The model under review builds one solid part; all positions refer to its coordinate system, in mm. A direction names the side the tool comes from. Round coordinates to 2 decimals unless told otherwise and drop trailing zeros. Write each loop counter-clockwise with the first axis right and the second up, starting at its lowest first coordinate (ties: lowest second). Pieces come first, ordered by that corner, then holes. Notation, with made-up numbers: (38, 45.25) -> (75, 45.25) arc R8 ccw to (75, 52.25) -> close; hole circle Ø7 at (25.25, 28.25). An arc over 180 degrees is marked (long way). Answer in a Markdown table with one row per item. Add a question column.
```python
from build123d import *

# Parameters (mm, degrees)
F0_W      = 77
F0_H      = 91
F0_W_2    = 50
F0_H_2    = 85
F1_DEPTH  = 3.1
F2_W      = 77
F2_H      = 91
F2_W_2    = 71
F2_H_2    = 85
F3_DEPTH  = 5
F4_W      = 3
F4_H      = 91
F5_DEPTH  = 25
F6_W      = 77
F6_H      = 91
F6_W_2    = 71
F6_H_2    = 85
F7_DEPTH  = 70
F9_DEPTH  = 91
F11_DEPTH = 77
F12_W     = 6
F12_H     = 8.1
F13_DEPTH = 4
F15_DEPTH = 91
F16_W     = 3
F16_H     = 91
F17_DEPTH = 25
F18_R     = 3


with BuildPart() as f1:
    # F0 (on Top) → F1 (new body)
    with BuildSketch(Plane.XY):
        Rectangle(F0_W, F0_H)
        Rectangle(F0_W_2, F0_H_2, mode=Mode.SUBTRACT)
    extrude(amount=F1_DEPTH)

    # F2 (on face) → F3 (join)
    with BuildSketch(Plane.XY.offset(3.1)):
        Rectangle(F2_W, F2_H)
        Rectangle(F2_W_2, F2_H_2, mode=Mode.SUBTRACT)
    extrude(amount=F3_DEPTH)

    # F4 (on face) → F5 (join)
    with BuildSketch(Plane.XY.offset(8.1)):
        with Locations((-37, 0)):
            Rectangle(F4_W, F4_H)
        with Locations((37, 0)):
            Rectangle(F4_W, F4_H)
    extrude(amount=F5_DEPTH)

    # F6 (on face) → F7 (join)
    with BuildSketch(Plane(origin=(0, 0, 0), x_dir=(1, 0, 0), z_dir=(0, 0, -1))):
        Rectangle(F6_W, F6_H)
        Rectangle(F6_W_2, F6_H_2, mode=Mode.SUBTRACT)
    extrude(amount=F7_DEPTH)

    # F8 (on face) → F9 (join)
    with BuildSketch(Plane(origin=(0, 45.5, 0), x_dir=(-1, 0, 0), z_dir=(0, 1, 0))):
        Polygon((38.5, -70), (38.5, 0), (15, 0), (35.5, -70), align=None)
        Polygon((-15, 0), (-38.5, 0), (-38.5, -70), (-35.5, -70), align=None)
    extrude(amount=-F9_DEPTH)

    # F10 (on face) → F11 (join)
    with BuildSketch(Plane.YZ.offset(38.5)):
        Polygon((45.5, -70), (45.5, 0), (15, 0), (42.5, -70), align=None)
        Polygon((-15, 0), (-45.5, 0), (-45.5, -70), (-42.5, -70), align=None)
    extrude(amount=-F11_DEPTH)

    # F12 (on face) → F13 (cut)
    with BuildSketch(Plane(origin=(0, -42.5, 0), x_dir=(-1, 0, 0), z_dir=(0, 1, 0))):
        with Locations((22, 4.05)):
            Rectangle(F12_W, F12_H)
    extrude(amount=-F13_DEPTH, mode=Mode.SUBTRACT)

    # F14 (on face) → F15 (join)
    with BuildSketch(Plane.XZ.offset(45.5)):
        Polygon((58.5, -70), (38.5, 33.1), (38.5, -70), align=None)
    extrude(amount=-F15_DEPTH)

    # F16 (on face) → F17 (cut)
    with BuildSketch(Plane.XY.offset(33.1)):
        with Locations((-37, 0)):
            Rectangle(F16_W, F16_H)
    extrude(amount=-F17_DEPTH, mode=Mode.SUBTRACT)

    # F18
    f18_edges = [f1.edges().sort_by_distance(p)[0] for p in [
        (-38.5, -45.5, -30.95),
        (-38.5, 45.5, -30.95),
    ]]
    fillet(f18_edges, radius=F18_R)


solid = f1.part
```
1. Add section A-A on y = -1. Write out the cut boundary in (x, z), plus the area to 3 significant figures.
2. Tool access review of faces 4 (the flat face through (-25, -1, 2)), 5 (the flat face through (30, 1, 3.1)), 6 (the flat face through (-27.384, 0.595, -42.288)), 7 (the flat face through (8, -44, 8.1)): name each direction out of +Z, -Z, +X, -X, +Y, -Y from which nothing blocks a thin tool from reaching the whole face with its end or side.
3. Add section B-B on x = -5.5. Write out the cut boundary in (y, z), plus the area to 3 significant figures.
4. Add section C-C on z = -9.5. Write out the cut boundary in (x, y).
5. Insertion check: pin 1 Ø9 at (y, z) = (17, 16.5) entering from -X; pin 2 Ø3 at (x, y) = (-31, 2.5) entering from +Z; pin 3 Ø10 at (y, z) = (-4, -16) entering from +X. Each pin has a flat end and moves straight along its axis. Give the tip position at first contact, or say it passes through.
6. Mouldability with a two-part tool opening along X and no side actions: class faces 1 (the flat face through (0.5, -32, -43.27)), 2 (the cylindrical face through (-37.64, -44.6, -30.4)), 3 (the flat face through (-37, 17, 8.1)) as pulls with the +X half, pulls with the -X half, needs draft (parallel to the pull), parting line crosses it, or undercut.
7. For L1, parallel to X at y = 15.5, z = -26; L2, parallel to Y at x = 3, z = -6; L3, parallel to X at y = 14.5, z = -17, list the stretches that pass through material, from the lowest coordinate up.
8. Add section D-D on x = 23. Write out the cut boundary in (y, z), plus the area to 3 significant figures.
Filled in:
| question | item | result |
|---|---|---|
| 1 | outline | (-38.5, -70) -> (-35.5, -70) -> (-15, 0) -> (-25, 0) -> (-25, 3.1) -> (-35.5, 3.1) -> (-35.5, 8.1) -> (-38.5, 8.1) -> close; (15, 0) -> (35.5, -70) -> (58.5, -70) -> (38.5, 33.1) -> (35.5, 33.1) -> (35.5, 3.1) -> (25, 3.1) -> (25, 0) -> close |
| 1 | area | 3,070 mm² |
| 2 | face 4 | +Z, -Y |
| 2 | face 5 | +Z |
| 2 | face 6 | -Z |
| 2 | face 7 | +Z, -X, +Y, -Y |
| 3 | outline | (-45.5, -70) -> (-42.5, -70) -> (-15, 0) -> (-42.5, 0) -> (-42.5, 8.1) -> (-45.5, 8.1) -> close; (15, 0) -> (42.5, -70) -> (45.5, -70) -> (45.5, 8.1) -> (42.5, 8.1) -> (42.5, 0) -> close |
| 3 | area | 2,390 mm² |
| 4 | outline | (-38.5, -42.5) arc R3 ccw to (-35.5, -45.5) -> (46.76, -45.5) -> (46.76, 45.5) -> (-35.5, 45.5) arc R3 ccw to (-38.5, 42.5) -> close; hole (-17.78, -18.73) -> (17.78, -18.73) -> (17.78, 18.73) -> (-17.78, 18.73) -> close |
| 5 | pin 1 | x = 35.5 |
| 5 | pin 2 | z = 3.1 |
| 5 | pin 3 | x = 48.99 |
| 6 | face 1 | undercut |
| 6 | face 2 | pulls with the -X half |
| 6 | face 3 | needs draft |
| 7 | L1 | -38.5 to -22.61, 22.61 to 49.96 |
| 7 | L2 | -45.5 to -17.36, 17.36 to 45.5 |
| 7 | L3 | -38.5 to -19.98, 19.98 to 48.22 |
| 8 | outline | (-45.5, -70) -> (-42.5, -70) -> (-25.73, -27.32) -> (25.73, -27.32) -> (42.5, -70) -> (45.5, -70) -> (45.5, 8.1) -> (42.5, 8.1) -> (42.5, 0) -> (-42.5, 0) -> (-42.5, 8.1) -> (-45.5, 8.1) -> close |
| 8 | area | 3,510 mm² |
